from build123d import *

# Parameters (mm, degrees)
F0_R     = 9
F0_R_2   = 7
F1_DEPTH = 5
F2_DEPTH = 10
F3_R     = 3
F4_DEPTH = 8


with BuildPart() as f1:
    # F0 (on Top) → F1 (new body)
    with BuildSketch(Plane.XY):
        Circle(F0_R)
        Circle(F0_R_2, mode=Mode.SUBTRACT)
        Circle(F0_R_2)
    extrude(amount=-F1_DEPTH)

    # F0 (on Top) → F2 (join)
    with BuildSketch(Plane.XY):
        Circle(F0_R_2)
    extrude(amount=F2_DEPTH)

    # F3 (on face) → F4 (cut)
    with BuildSketch(Plane.XY.offset(10)):
        Circle(F3_R)
    extrude(amount=-F4_DEPTH, mode=Mode.SUBTRACT)


solid = f1.part
Design review of the part built by this model. Coordinates are the model's own, in mm. A direction names the side the tool comes from. Coordinates: 2 decimals unless noted, no trailing zeros. Loops run counter-clockwise (first coordinate to the right, second up) from the corner with the lowest first, then second, coordinate; pieces in that order, holes last. Notation, with made-up numbers: (53, 19) -> (104, 19) arc R6 cw to (104, 23) -> close; hole circle Ø5 at (39.25, 55). An arc over 180 degrees is marked (long way). Use a Markdown table: item, result. Add a question column.
Item 1: We need section A-A, the plane y = 0. Write out the cut boundary in (x, z), and give its area (3 significant figures).
Item 2: Wall thickness on L1, parallel to Y at x = 0, z = 5.25; L2, parallel to Z at x = 2.75, y = 7.5; L3, parallel to Y at x = 2, z = 8: over which ranges is each line inside the solid? List them lowest first. Write a range as from..to.
Item 3: The part is to be moulded in two halves that separate along Y. For faces 1 (the flat face through (0, 0, 2)), 2 (the cylindrical face through (6.466, -2.681, 4.93)), 3 (the flat face through (0, 0, -5)), say which applies: +Y half, -Y half, draft (parallel to the pull), parting line (faces both ways), or undercut.
Item 4: We need section C-C, the plane z = 1. Write out the cut boundary in (x, y).
Item 5: Machinability: for faces 4 (the flat face through (0, -7.3, 0)), 5 (the cylindrical face through (-1.172, 8.923, -2.465)), which of the approach directions +Z, -Z, +X, -X, +Y, -Y give a long, thin tool a straight path to every point of the face, cutting with its end or side? Answer none if there is none.
Item 6: Clearance check with flat-ended pins moving along their axes: P1, Ø2, axis at y = 3.5, z = -1.5, coming from the -X side; P2, Ø6, axis at y = -3, z = 4.5, coming from the +X side; P3, Ø8, axis at y = -5.5, z = 0.5, coming from the -X side. State where each tip first meets the part, or that it passes through.
Item 7: We need section D-D, the plane z = 2.5. Write out the cut boundary in (x, y).
Numbers:
| question | item | result |
|---|---|---|
| 1 | outline | (-9, -5) -> (9, -5) -> (9, 0) -> (7, 0) -> (7, 10) -> (3, 10) -> (3, 2) -> (-3, 2) -> (-3, 10) -> (-7, 10) -> (-7, 0) -> (-9, 0) -> close |
| 1 | area | 182 mm^2 |
| 2 | L1 | y = -7..-3, 3..7 |
| 2 | L2 | z = -5..0 |
| 2 | L3 | y = -6.71..-2.24, 2.24..6.71 |
| 3 | face 1 | undercut |
| 3 | face 2 | parting line |
| 3 | face 3 | draft |
| 4 | outline | circle Ø14 at (0, 0) |
| 5 | face 4 | +Z |
| 5 | face 5 | +Z, -Z |
| 6 | P1 | stops at x = -8.65 |
| 6 | P2 | stops at x = 7 |
| 6 | P3 | stops at x = -8.87 |
| 7 | outline | circle Ø14 at (0, 0); hole circle Ø6 at (0, 0) |
